Design review of the part built by this model. Coordinates are the model's own, in mm. A direction names the side the tool comes from. Coordinates: 2 decimals unless noted, no trailing zeros. Write each loop counter-clockwise with the first axis right and the second up, starting at its lowest first coordinate (ties: lowest second). Pieces come first, ordered by that corner, then holes.
Q1. Clearance check with flat-ended pins moving along their axes: pin 1 Ø4 at (x, y) = (3.5, 1.5) entering from -Z; pin 2 Ø0.6 at (y, z) = (4.5, 11.5) entering from -X. State where each tip first meets the part, or that it passes through.
Q2. Add section D-D, the plane x = 4. Give the boundary of the cut face in (y, z) (3 decimals).
Q3. Add section A-A, the plane z = 4. Give the boundary of the cut face in (x, y) (3 decimals).
Q4. Machinability: for faces 1 (the face through (2, 6, 12)), 2 (the face through (2.73, 3.47, 4.44)), 3 (the face through (4, 4, 14)), which of the approach directions +Z, -Z, +X, -X, +Y, -Y give a long, thin tool a straight path to every point of the face, cutting with its end or side? Answer none if there is none.
Q5. To check wall thickness, follow probe 1 along Z at (x, y) = (2.25, 4); probe 2 along Y at (x, z) = (4, 4) (3 decimals); probe 3 along Y at (x, z) = (4, 11). State the ranges of each line that lie inside material, in increasing order.
Q6. Add section C-C, the plane y = 4. Give the boundary of the cut face in (x, z) (3 decimals).
Q7. The part is to be moulded in two halves that separate along Z. For faces 4 (the face through (0, 4, 7)), 5 (the face through (6, 4, 0)), 6 (the face through (5, 6, 11)), say which applies: +Z half, -Z half, draft (parallel to the pull), parting line (faces both ways), or undercut.
Q8. Add section B-B, the plane x = 0.5. Give the boundary of the cut face in (y, z), plus the area to 3 significant figures.
from build123d import *

# Parameters (mm, degrees)
SZKIC1_W                    = 8
SZKIC1_H                    = 8
DODANIE_WYCI_GNI_CIE1_DEPTH = 14
SZKIC2_W                    = 5
SZKIC2_H                    = 2
WYTNIJ_WYCI_GNI_CIE1_DEPTH  = 5
SZKIC3_R                    = 1.375
WYTNIJ_WYCI_GNI_CIE2_DEPTH  = 9


with BuildPart() as part:
    # Szkic1 → Dodanie-wyciągnięcie1 (new body)
    with BuildSketch(Plane.XY):
        with Locations((4, 4)):
            Rectangle(SZKIC1_W, SZKIC1_H)
    extrude(amount=DODANIE_WYCI_GNI_CIE1_DEPTH)

    # Szkic2 → Wytnij-wyciągnięcie1 (cut)
    with BuildSketch(Plane(origin=(0, 8, 0), x_dir=(1, 0, 0), z_dir=(0, 1, 0))):
        with Locations((2.5, -11)):
            Rectangle(SZKIC2_W, SZKIC2_H)
    extrude(amount=-WYTNIJ_WYCI_GNI_CIE1_DEPTH, mode=Mode.SUBTRACT)

    # Szkic3 → Wytnij-wyciągnięcie2 (cut)
    with BuildSketch(Plane(origin=(0, 0, 0), x_dir=(-1, 0, 0), z_dir=(0, 0, -1))):
        with Locations((-4, 4)):
            Circle(SZKIC3_R)
    extrude(amount=-WYTNIJ_WYCI_GNI_CIE2_DEPTH, mode=Mode.SUBTRACT)


solid = part.part
Here are the results:
1. pin 1: stops at z = 0
1. pin 2: stops at x = 5
2. outline: (0, 0) - (2.625, 0) - (2.625, 9) - (5.375, 9) - (5.375, 0) - (8, 0) - (8, 10) - (3, 10) - (3, 12) - (8, 12) - (8, 14) - (0, 14) - close
3. outline: (0, 0) - (8, 0) - (8, 8) - (0, 8) - close; hole circle Ø2.75 at (4, 4)
4. face 1: -X, +Y
4. face 2: -Z
4. face 3: +Z, +X, -X, +Y, -Y
5. probe 1: z = 0 to 10, 12 to 14
5. probe 2: y = 0 to 2.625, 5.375 to 8
5. probe 3: y = 0 to 3
6. outline: (0, 0) - (2.625, 0) - (2.625, 9) - (5.375, 9) - (5.375, 0) - (8, 0) - (8, 14) - (0, 14) - (0, 12) - (5, 12) - (5, 10) - (0, 10) - close
7. face 4: draft
7. face 5: -Z half
7. face 6: undercut
8. outline: (0, 0) - (8, 0) - (8, 10) - (3, 10) - (3, 12) - (8, 12) - (8, 14) - (0, 14) - close
8. area: 102 mm2
